```python
from build123d import *

# Parameters (mm, degrees)
F0_R     = 47.5
F0_R_2   = 41.5
F1_DEPTH = 16
F2_DEPTH = 1.2
F3_SIZE  = 2
F4_R     = 48.436615
F4_R_2   = 47.5
F4_R_3   = 45.5
F5_DEPTH = 8


# Not quite as in the source:
# - a fillet or chamfer that OpenCascade refuses, or shapes differently, is made with other operations: its cross-section is extruded or revolved along the edge and cut away or added


with BuildPart() as f1:
    # F0 (on Top) → F1 (new body)
    with BuildSketch(Plane.XY):
        Circle(F0_R)
        Circle(F0_R_2, mode=Mode.SUBTRACT)
    extrude(amount=F1_DEPTH)

    # F0 (on Top) → F2 (join)
    with BuildSketch(Plane.XY):
        Circle(F0_R_2)
    extrude(amount=F2_DEPTH)

    # F3
    f3_edges = [f1.edges().sort_by_distance(p)[0] for p in [
        (-41.5, 0, 16),
    ]]
    chamfer(f3_edges, length=F3_SIZE)

    # F4 (on face) → F5 (cut, symmetric)
    with BuildSketch(Plane(origin=(0, 0, 0), x_dir=(1, 0, 0), z_dir=(0, 0, -1))):
        Circle(F4_R)
        Circle(F4_R_2, mode=Mode.SUBTRACT)
        Circle(F4_R_2)
        Circle(F4_R_3, mode=Mode.SUBTRACT)
    extrude(amount=F5_DEPTH, both=True, mode=Mode.SUBTRACT)

    # F6: fillet of radius 4 on 2 edges, made by hand

    # F6_s1 → F6_t2 (revolve, cut)
    with BuildSketch(Plane.XZ):
        with BuildLine():
            ThreePointArc((47.5, 11.4641016151), (46.9641016151, 9.4641016151), (45.5, 8))
            Line((45.5, 8), (47.5, 8))
            Line((47.5, 8), (47.5, 11.4641016151))
        make_face()
    revolve(axis=Axis((0, 0, 8), (0, 0, -1)), mode=Mode.SUBTRACT)

    # F6_s3 → F6_t4 (revolve, cut)
    with BuildSketch(Plane.XZ):
        with BuildLine():
            ThreePointArc((45.5, 4), (44.3284271247, 1.1715728753), (41.5, 0))
            Line((41.5, 0), (45.5, 0))
            Line((45.5, 0), (45.5, 4))
        make_face()
    revolve(axis=Axis((0, 0, 0), (0, 0, 1)), mode=Mode.SUBTRACT)


solid = f1.part
```
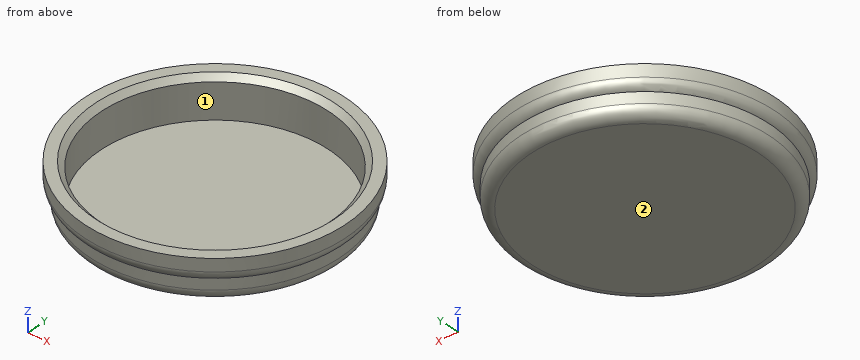
Verification items for the finished model (mm, model axes). Face numbers are marked on the shaded views. Give positions to 0.01 mm unless a question says otherwise; leave off trailing zeros. Order: outer loops, then holes, each group sorted by start corner. A loop starts at its lowest first (then second) coordinate and runs counter-clockwise, first axis right, second up. Notation, with made-up numbers: (-24.5, -23) -> (-8.5, -23) arc R23 ccw to (-8.5, -8) -> close; hole circle Ø4 at (71, -15.5). An arc over 180 degrees is marked (long way). Use a Markdown table: item, result.
1) Material ranges on probe 1 along Y at (x, z) = (0, 7.75); probe 2 along Z at (x, y) = (17, -18); probe 3 along Y at (x, z) = (35.5, 13), recorded low to high.
Results:
| item | result |
|---|---|
| probe 1 | -45.5 to -41.5, 41.5 to 45.5 |
| probe 2 | 0 to 1.2 |
| probe 3 | -31.56 to -21.49, 21.49 to 31.56 |
2) Section check C-C, the plane z = 2.75. Record the boundary of the cut face in (x, y), then the cut area to 3 significant figures.
Results:
| item | result |
|---|---|
| outline | circle Ø90.6 at (0, 0); hole circle Ø83 at (0, 0) |
| area | 1,040 mm² |
3) Depth check by flat-ended pin: pin 1 Ø4 at (y, z) = (-19, 3) entering from +X; pin 2 Ø4 at (x, y) = (33, 11) entering from +Z; pin 3 Ø8 at (x, z) = (24, 13) entering from +Y; pin 4 Ø3 at (x, y) = (-28, -12.5) entering from -Z. Enter the tip coordinate at first touch or a pass-through.
Results:
| item | result |
|---|---|
| pin 1 | x = 42.15 |
| pin 2 | z = 1.2 |
| pin 3 | y = 43.08 |
| pin 4 | z = 0 |
4) Mould release check, pull along X, two halves, no side actions. Record for the marked faces 1 and 2: pulls with the +X half, pulls with the -X half, needs draft (parallel to the pull), parting line crosses it, or undercut.
Results:
| item | result |
|---|---|
| face 1 | undercut |
| face 2 | needs draft |
5) Section check A-A, the plane x = 0. Record the boundary of the cut face in (y, z), then the cut area to 3 significant figures.
Results:
| item | result |
|---|---|
| outline | (-47.5, 11.46) arc R4 ccw to (-45.5, 8) -> (-45.5, 4) arc R4 ccw to (-41.5, 0) -> (41.5, 0) arc R4 ccw to (45.5, 4) -> (45.5, 8) arc R4 ccw to (47.5, 11.46) -> (47.5, 16) -> (43.5, 16) -> (41.5, 14) -> (41.5, 1.2) -> (-41.5, 1.2) -> (-41.5, 14) -> (-43.5, 16) -> (-47.5, 16) -> close |
| area | 245 mm² |
